Can you work these out from the model? Positions are in its coordinate system, mm. Face numbers are marked on the shaded views. A direction names the side the tool comes from. Round coordinates to 2 decimals unless told otherwise and drop trailing zeros. Write each loop counter-clockwise with the first axis right and the second up, starting at its lowest first coordinate (ties: lowest second). Pieces come first, ordered by that corner, then holes.
Q1. If we section it at B-B (z = 3.75): Please give me the cut outline in (x, y).
Q2. For the marked faces 1 and 2, which set-ups out of +Z, -Z, +X, -X, +Y, -Y let a thin tool reach every point of the face, with its end or its side?
Q3. Please list where these lines run through material, in increasing order: line 1 along X through (y, z) = (0.25, -1.75); line 2 along Y through (x, z) = (-6, -5); line 3 along Z through (x, y) = (16, 4.25).
Q4. If we section it at C-C (x = 14): Please give me the cut outline in (y, z).
Q5. If we section it at A-A (y = 6): Please give me the cut outline in (x, z).
Q6. If we section it at D-D (y = 0.5): Please give me the cut outline in (x, z).
Q7. I'm going to push flat-ended pins straight in: pin 1 Ø6 at (x, z) = (-15, -4.5) entering from -Y; pin 2 Ø2 at (x, z) = (-15, -2.5) entering from +Y; pin 3 Ø6 at (x, z) = (4, -5) entering from -Y. Where does each tip first touch, or does it pass through?
from build123d import *

# Parameters (mm, degrees)
F0_W        = 40
F0_H        = 10
F2_DEPTH    = 5
F3_ANGLE    = 45
F5_DEPTH    = 12.5
F6_T4_DEPTH = 15.1421356237
F7_T4_DEPTH = 15.1421356237


# Not quite as in the source:
# - a fillet or chamfer that OpenCascade refuses, or shapes differently, is made with other operations: its cross-section is extruded or revolved along the edge and cut away or added
# - a feature names something its author has since deleted; it is built from what else it names


with BuildPart() as f2:
    # F0 (on Top) → F2 (new body, symmetric)
    with BuildSketch(Plane.XY):
        Rectangle(F0_W, F0_H)
    extrude(amount=F2_DEPTH, both=True)


with BuildPart() as f2_1:
    # F3: moved
    add(f2.part.rotate(Axis((0, 0, 0), (-1, 0, 0)), F3_ANGLE))

    # F4 (on offset) → F5 (cut, symmetric)
    with BuildSketch(Plane.XY.offset(5)):
        Polygon((-0.8578643763, 7.0710678119), (-15, 7.0710678119), (-7.9289321881, 0), align=None)
        Polygon((15.5842712475, 7.0710678119), (1.4421356237, 7.0710678119), (8.5132034356, 0), align=None)
    extrude(amount=F5_DEPTH, both=True, mode=Mode.SUBTRACT)

    # F6: fillet of radius 0.2 on 1 edges, made by hand


with BuildPart() as f6_tool2:
    # F6_s3 → F6_t4 (new body)
    with BuildSketch(Plane.XY.offset(7.5710678119)):
        with BuildLine():
            ThreePointArc((-8.0703535444, 0.1414213562), (-7.9289321881, 0.0828427125), (-7.7875108319, 0.1414213562))
            Line((-7.7875108319, 0.1414213562), (-7.9289321881, 0))
            Line((-7.9289321881, 0), (-8.0703535444, 0.1414213562))
        make_face()
    extrude(amount=-F6_T4_DEPTH)

    split(bisect_by=Plane(origin=(0, 3.5355339059, 3.5355339059), x_dir=(1, 0, 0), z_dir=(0, -0.7071067812, -0.7071067812)), keep=Keep.TOP)

    split(bisect_by=Plane(origin=(0, 3.5355339059, -3.5355339059), x_dir=(1, 0, 0), z_dir=(0, -0.7071067812, 0.7071067812)), keep=Keep.TOP)


with BuildPart() as f2_2:
    add(f2_1.part)

    # F6_t1: union F6_tool2
    add(f6_tool2.part)

    # F7: fillet of radius 0.2 on 1 edges, made by hand


with BuildPart() as f7_tool2:
    # F7_s3 → F7_t4 (new body)
    with BuildSketch(Plane.XY.offset(7.5710678119)):
        with BuildLine():
            ThreePointArc((8.3717820794, 0.1414213562), (8.5132034356, 0.0828427125), (8.6546247918, 0.1414213562))
            Line((8.6546247918, 0.1414213562), (8.5132034356, 0))
            Line((8.5132034356, 0), (8.3717820794, 0.1414213562))
        make_face()
    extrude(amount=-F7_T4_DEPTH)

    split(bisect_by=Plane(origin=(0, 3.5355339059, -3.5355339059), x_dir=(1, 0, 0), z_dir=(0, -0.7071067812, 0.7071067812)), keep=Keep.TOP)

    split(bisect_by=Plane(origin=(0, 3.5355339059, 3.5355339059), x_dir=(1, 0, 0), z_dir=(0, -0.7071067812, -0.7071067812)), keep=Keep.TOP)


with BuildPart() as f2_3:
    add(f2_2.part)

    # F7_t1: union F7_tool2
    add(f7_tool2.part)


solid = f2_3.part
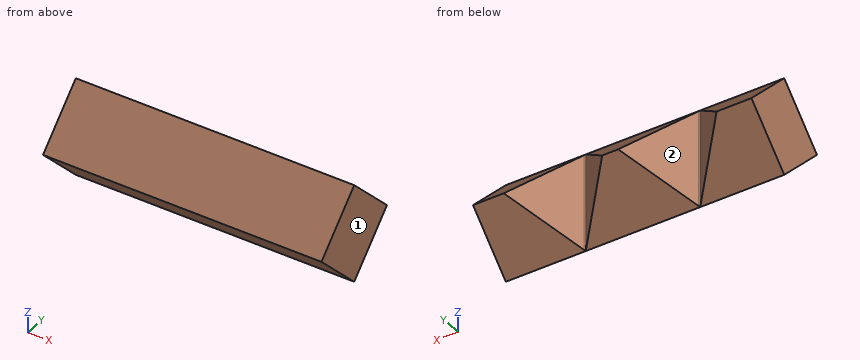
A:
1. outline: (-20, -3.32) - (20, -3.32) - (20, 3.32) - (11.83, 3.32) - (8.65, 0.14) arc R0.2 cw to (8.37, 0.14) - (5.19, 3.32) - (-4.61, 3.32) - (-7.79, 0.14) arc R0.2 cw to (-8.07, 0.14) - (-11.25, 3.32) - (-20, 3.32) - close
2. face 1: +Z, -Z, +X, +Y, -Y
2. face 2: +Z, -Z, +Y
3. line 1: x = -20 to -8.18, -7.68 to 8.26, 8.76 to 20
3. line 2: y = -2.07 to 1.93
3. line 3: z = -2.82 to 2.82
4. outline: (-7.07, 0) - (0, -7.07) - (5.49, -1.58) - (5.49, 1.58) - (0, 7.07) - close
5. outline: (-20, -1.07) - (-13.93, -1.07) - (-13.93, 1.07) - (-20, 1.07) - close; (-1.93, -1.07) - (2.51, -1.07) - (2.51, 1.07) - (-1.93, 1.07) - close; (14.51, -1.07) - (20, -1.07) - (20, 1.07) - (14.51, 1.07) - close
6. outline: (-20, -6.57) - (-8.43, -6.57) - (-8.43, 6.57) - (-20, 6.57) - close; (-7.43, -6.57) - (8.01, -6.57) - (8.01, 6.57) - (-7.43, 6.57) - close; (9.01, -6.57) - (20, -6.57) - (20, 6.57) - (9.01, 6.57) - close
7. pin 1: stops at y = -5.57
7. pin 2: stops at y = 5.57
7. pin 3: stops at y = -5.07
